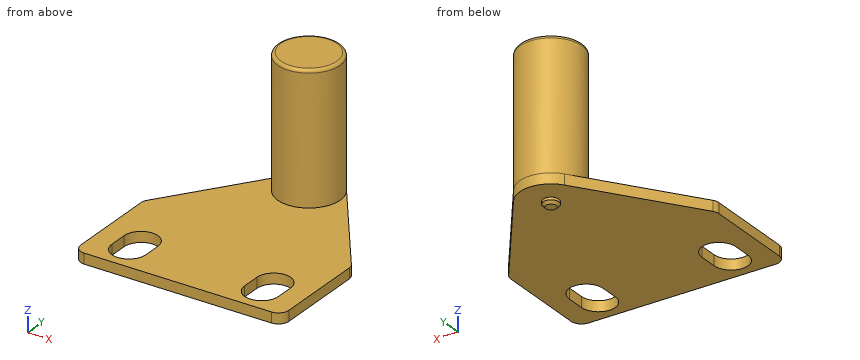
from build123d import *

# Parameters (mm, degrees)
PAD_DEPTH    = 2
SKETCH001_R  = 6
PAD001_DEPTH = 25
SKETCH002_R  = 1.5
PAD002_DEPTH = 1
FILLET_R     = 2
FILLET001_R  = 0.6
CHAMFER_SIZE = 0.5


with BuildPart() as part:
    # Sketch → Pad (new body)
    with BuildSketch(Plane.XY):
        with BuildLine():
            Line((-20, 0), (20, 0))
            Line((20, 0), (20, 20))
            Line((20, 20), (4.882401, 41.164639))
            ThreePointArc((4.882401, 41.164639), (0, 43.67721), (-4.882401, 41.164639))
            Line((-4.882401, 41.164639), (-20, 20))
            Line((-20, 20), (-20, 0))
        make_face()
        with BuildLine():
            ThreePointArc((16, 8.5), (12.75, 11.75), (9.5, 8.5))
            Line((9.5, 8.5), (9.5, 5))
            ThreePointArc((9.5, 5), (12.75, 1.75), (16, 5))
            Line((16, 8.5), (16, 5))
        make_face(mode=Mode.SUBTRACT)
        with BuildLine():
            ThreePointArc((-9.5, 8.5), (-12.75, 11.75), (-16, 8.5))
            Line((-16, 8.5), (-16, 5))
            ThreePointArc((-16, 5), (-12.75, 1.75), (-9.5, 5))
            Line((-9.5, 8.5), (-9.5, 5))
        make_face(mode=Mode.SUBTRACT)
    extrude(amount=PAD_DEPTH)

    # Sketch001 (on Face16 of Pad) → Pad001 (join)
    with BuildSketch(Plane.XY.offset(2)):
        with Locations((0, 37.67721)):
            Circle(SKETCH001_R)
    extrude(amount=PAD001_DEPTH)

    # Sketch002 (on Face4 of Pad001) → Pad002 (join)
    with BuildSketch(Plane(origin=(0, 0, 0), x_dir=(1, 0, 0), z_dir=(0, 0, -1))):
        with Locations((0, -37.67721)):
            Circle(SKETCH002_R)
    extrude(amount=PAD002_DEPTH)

    # Fillet
    fillet_edges = [part.edges().sort_by_distance(p)[0] for p in [
        (20, 0, 1),
        (-20, 0, 1),
        (-20, 20, 1),
        (20, 20, 1),
    ]]
    fillet(fillet_edges, radius=FILLET_R)

    # Fillet001
    fillet001_edges = [part.edges().sort_by_distance(p)[0] for p in [
        (-6, 37.67721, 27),
    ]]
    fillet(fillet001_edges, radius=FILLET001_R)

    # Chamfer
    chamfer_edges = [part.edges().sort_by_distance(p)[0] for p in [
        (-1.5, 37.67721, -1),
    ]]
    chamfer(chamfer_edges, length=CHAMFER_SIZE)


solid = part.part
Here's how the part is built. I have some questions about the finished solid (model axes, mm). Round coordinates to 2 decimals unless told otherwise and drop trailing zeros. Write each loop counter-clockwise with the first axis right and the second up, starting at its lowest first coordinate (ties: lowest second). Pieces come first, ordered by that corner, then holes.
1. Suppose I cut it at B-B (z = 1). List the corners of the cut face in (x, y) for me.
2. Will these pins go through, and if not, where does the flat tip stop? pin 1 Ø12 at (x, y) = (3.5, 14.5) entering from +Z; pin 2 Ø10 at (x, y) = (-14.5, 12) entering from -Z; pin 3 Ø12 at (y, z) = (34, 8.5) entering from -X.
3. Suppose I cut it at D-D (y = 23.5). List the corners of the cut face in (x, z) for me.
4. I need wall thicknesses on L1, parallel to Z at x = 0.5, y = 22.5; L2, parallel to Z at x = 5, y = 40; L3, parallel to X at y = 34.5, z = 10.25. Which ranges of each line are inside material? Lowest first, please.
5. Suppose I cut it at C-C (x = 0). List the corners of the cut face in (y, z) for me.
6. Suppose I cut it at A-A (x = 14). List the corners of the cut face in (y, z) for me.
Answer sheet:
1. outline: (-20, 2) arc R2 ccw to (-18, 0) - (18, 0) arc R2 ccw to (20, 2) - (20, 19.36) arc R2 ccw to (19.63, 20.52) - (4.88, 41.16) arc R6 ccw to (-4.88, 41.16) - (-19.63, 20.52) arc R2 ccw to (-20, 19.36) - close; hole (-16, 5) arc R3.25 ccw to (-9.5, 5) - (-9.5, 8.5) arc R3.25 ccw to (-16, 8.5) - close; hole (9.5, 5) arc R3.25 ccw to (16, 5) - (16, 8.5) arc R3.25 ccw to (9.5, 8.5) - close
2. pin 1: stops at z = 2
2. pin 2: stops at z = 0
2. pin 3: stops at x = -6
3. outline: (-17.5, 0) - (17.5, 0) - (17.5, 2) - (-17.5, 2) - close
4. L1: z = 0 to 2
4. L2: z = 0 to 26.99
4. L3: x = -5.09 to 5.09
5. outline: (0, 0) - (36.18, 0) - (36.18, -0.5) - (36.68, -1) - (38.68, -1) - (39.18, -0.5) - (39.18, 0) - (43.68, 0) - (43.68, 26.4) arc R0.6 ccw to (43.08, 27) - (32.28, 27) arc R0.6 ccw to (31.68, 26.4) - (31.68, 2) - (0, 2) - close
6. outline: (0, 0) - (2, 0) - (2, 2) - (0, 2) - close; (11.5, 0) - (28.4, 0) - (28.4, 2) - (11.5, 2) - close
